Geometry: final body of the model. Coordinates: model frame, mm. A direction names the side the tool comes from. Coordinates: 2 decimals unless noted, no trailing zeros. Loops run counter-clockwise (first coordinate to the right, second up) from the corner with the lowest first, then second, coordinate; pieces in that order, holes last. Notation, with made-up numbers: (33.25, 41) -> (92.25, 41) arc R17 cw to (92.25, 64) -> close; hole circle Ø1 at (-27, 34.25). An arc over 180 degrees is marked (long way). One line per item, written item: value. Start each with the question number.
Item 1: Contact query for flat-ended pins moving along their axis: pin 1 Ø13 at (x, y) = (163.5, 44) entering from -Z; pin 2 Ø21 at (x, z) = (392.5, -577.5) entering from +Y; pin 3 Ø21.5 at (x, z) = (218, 289) entering from +Y; pin 4 Ø21 at (x, y) = (384, 408) entering from +Z. Output: stop coordinate, or through.
Item 2: Section query C-C on z = 231.5. Return loops of the section in (x, y).
Item 3: Section query B-B on z = -418. Return loops of the section in (x, y), then the cut area to 3 significant figures.
Item 4: Set-up query: faces 5 (the flat face through (198, 404, -399.91)), 6 (the flat face through (11, 387.823, 144)), 7 (the flat face through (11, 49, 99.89)), 8 (the flat face through (12, 394.98, -375)), 9 (the flat face through (198, 394.98, -259)). Return all of +Z, -Z, +X, -X, +Y, -Y with unobstructed straight access to the full face (end or side cutting, diameter ignored); none if empty.
Item 5: Mould query, pull axis X, two halves, no side actions, for faces 1 (the flat face through (402, 405, -259)), 2 (the flat face through (389, 414.065, -501)), 3 (the flat face through (342.591, 227, 120)), 4 (the flat face through (198, 35.935, 122)). Classes: +X half, -X half, draft (parallel to the pull), parting line (faces both ways), or undercut.
Item 6: Section query A-A on y = 313. Return loops of the section in (x, z) (3 decimals).
Item 7: Ray query, probe 1 along Z at (x, y) = (291, 55); probe 2 along Z at (x, y) = (364, 289) (3 decimals); probe 3 along X at (y, z) = (56, 244.5). Return the intervals inside material, ascending. Write a range as from..to.
Item 8: Section query D-D on x = 353.5. Return loops of the section in (y, z) (3 decimals), then the cut area to 3 significant figures.
from build123d import *

# Parameters (mm, degrees)
SKETCH2_W                       = 400
SKETCH2_H                       = 450
BOSS_EXTRUDE1_DEPTH             = 30
SKETCH3_W                       = 40
SKETCH3_H                       = 50
BOSS_EXTRUDE2_DEPTH             = 400
SKETCH4_W                       = 40
SKETCH4_H                       = 40
BOSS_EXTRUDE3_DEPTH             = 600
SKETCH5_W                       = 40.556580032
SKETCH5_H                       = 28.62817414
SKETCH5_W_2                     = 47.713623567
BOSS_EXTRUDE4_DEPTH             = 402
SKETCH6_W                       = 42.94226121
SKETCH6_H                       = 26.242492962
SKETCH6_W_2                     = 42.942261211
BOSS_EXTRUDE5_DEPTH             = 402
SKETCH7_W                       = 40.556580032
SKETCH7_H                       = 19.085449427
SKETCH7_W_2                     = 50.099304746
SKETCH7_W_3                     = 42.94226121
SKETCH7_W_4                     = 44.71367334
BOSS_EXTRUDE6_DEPTH             = 402
BOSS_EXTRUDE7_REACH             = 816.236
SKETCH8_W                       = 21.611464792
SKETCH8_H                       = 67.92174649
SKETCH8_H_2                     = 58.65969015
BOSS_EXTRUDE7_DIRECTION_2_DEPTH = 2
BOSS_EXTRUDE8_REACH             = 816.236
SKETCH9_W                       = 23.109912939
SKETCH9_H                       = 42.918409744
SKETCH9_H_2                     = 49.521242012


with BuildPart() as part:
    # Sketch2 → Boss-Extrude1 (new body)
    with BuildSketch(Plane.XY):
        with Locations((200, 225)):
            Rectangle(SKETCH2_W, SKETCH2_H)
    extrude(amount=BOSS_EXTRUDE1_DEPTH)

    # Sketch3 → Boss-Extrude2 (add)
    with BuildSketch(Plane.XY.offset(30)):
        with Locations((43, 401)):
            Rectangle(SKETCH3_W, SKETCH3_H)
        with Locations((357, 401)):
            Rectangle(SKETCH3_W, SKETCH3_H)
        with Locations((357, 49)):
            Rectangle(SKETCH3_W, SKETCH3_H)
        with Locations((43, 49)):
            Rectangle(SKETCH3_W, SKETCH3_H)
    extrude(amount=BOSS_EXTRUDE2_DEPTH)

    # Sketch4 → Boss-Extrude3 (add)
    with BuildSketch(Plane(origin=(0, 0, 0), x_dir=(-1, 0, 0), z_dir=(0, 0, -1))):
        with Locations((-356, 406)):
            Rectangle(SKETCH4_W, SKETCH4_H)
        with Locations((-44, 406)):
            Rectangle(SKETCH4_W, SKETCH4_H)
    extrude(amount=BOSS_EXTRUDE3_DEPTH)

    # Sketch5 → Boss-Extrude4 (add)
    with BuildSketch(Plane(origin=(0, 0, 0), x_dir=(0, 0, -1), z_dir=(1, 0, 0))):
        with Locations((-144.025393122, 402.136827493)):
            Rectangle(SKETCH5_W, SKETCH5_H)
        with Locations((-280.009220289, 402.136827493)):
            Rectangle(SKETCH5_W_2, SKETCH5_H)
    extrude(amount=BOSS_EXTRUDE4_DEPTH)

    # Sketch6 → Boss-Extrude5 (add)
    with BuildSketch(Plane(origin=(0, 0, 0), x_dir=(0, 0, -1), z_dir=(1, 0, 0))):
        with Locations((-280.009220288, 49.056013096)):
            Rectangle(SKETCH6_W, SKETCH6_H)
        with Locations((-121.361421928, 49.056013096)):
            Rectangle(SKETCH6_W_2, SKETCH6_H)
    extrude(amount=BOSS_EXTRUDE5_DEPTH)

    # Sketch7 → Boss-Extrude6 (add)
    with BuildSketch(Plane(origin=(0, 0, 0), x_dir=(0, 0, -1), z_dir=(1, 0, 0))):
        with Locations((259.15472602, 404.522508672)):
            Rectangle(SKETCH7_W, SKETCH7_H)
        with Locations((374.86026317, 404.522508672)):
            Rectangle(SKETCH7_W_2, SKETCH7_H)
        with Locations((501.301365623, 404.522508672)):
            Rectangle(SKETCH7_W_3, SKETCH7_H)
        with Locations((577.64316333, 404.522508672)):
            Rectangle(SKETCH7_W_4, SKETCH7_H)
    extrude(amount=BOSS_EXTRUDE6_DEPTH)

    # Sketch8 → Boss-Extrude7 (add, up to next)
    with BuildSketch(Plane(origin=(0, 74, 0), x_dir=(1, 0, 0), z_dir=(0, 1, 0)), mode=Mode.PRIVATE) as boss_extrude7_sk1:
        with Locations((41.856325516, -134.973838063)):
            Rectangle(SKETCH8_W, SKETCH8_H)
    boss_extrude7_tool1 = extrude(boss_extrude7_sk1.sketch, amount=BOSS_EXTRUDE7_REACH, mode=Mode.PRIVATE) - part.part
    # Sketch8 → Boss-Extrude7 (add, up to next)
    with BuildSketch(Plane(origin=(0, 74, 0), x_dir=(1, 0, 0), z_dir=(0, 1, 0)), mode=Mode.PRIVATE) as boss_extrude7_sk2:
        with Locations((41.856325516, -284.710415551)):
            Rectangle(SKETCH8_W, SKETCH8_H_2)
    boss_extrude7_tool2 = extrude(boss_extrude7_sk2.sketch, amount=BOSS_EXTRUDE7_REACH, mode=Mode.PRIVATE) - part.part
    add(boss_extrude7_tool1.solids().sort_by_distance((41.856326, 74, 134.973838))[0])
    add(boss_extrude7_tool2.solids().sort_by_distance((41.856326, 74, 284.710416))[0])

    # Sketch8 → Boss-Extrude7 direction 2 (add)
    with BuildSketch(Plane(origin=(0, 74, 0), x_dir=(1, 0, 0), z_dir=(0, 1, 0))):
        with Locations((41.856325516, -134.973838063)):
            Rectangle(SKETCH8_W, SKETCH8_H)
        with Locations((41.856325516, -284.710415551)):
            Rectangle(SKETCH8_W, SKETCH8_H_2)
    extrude(amount=-BOSS_EXTRUDE7_DIRECTION_2_DEPTH)

    # Sketch9 → Boss-Extrude8 (add, up to next)
    with BuildSketch(Plane.XZ.offset(-376), mode=Mode.PRIVATE) as boss_extrude8_sk1:
        with Locations((354.146322372, 280.024195097)):
            Rectangle(SKETCH9_W, SKETCH9_H)
    boss_extrude8_tool1 = extrude(boss_extrude8_sk1.sketch, amount=BOSS_EXTRUDE8_REACH, mode=Mode.PRIVATE) - part.part
    # Sketch9 → Boss-Extrude8 (add, up to next)
    with BuildSketch(Plane.XZ.offset(-376), mode=Mode.PRIVATE) as boss_extrude8_sk2:
        with Locations((354.146322372, 119.905512592)):
            Rectangle(SKETCH9_W, SKETCH9_H_2)
    boss_extrude8_tool2 = extrude(boss_extrude8_sk2.sketch, amount=BOSS_EXTRUDE8_REACH, mode=Mode.PRIVATE) - part.part
    add(boss_extrude8_tool1.solids().sort_by_distance((354.146322, 376, 280.024195))[0])
    add(boss_extrude8_tool2.solids().sort_by_distance((354.146322, 376, 119.905513))[0])


solid = part.part
Reply:
1. pin 1: stops at z = 0
1. pin 2: stops at y = 414.07
1. pin 3: stops at y = 416.45
1. pin 4: stops at z = 430
2. outline: (23, 24) -> (63, 24) -> (63, 74) -> (23, 74) -> close; (23, 376) -> (63, 376) -> (63, 426) -> (23, 426) -> close; (337, 24) -> (377, 24) -> (377, 74) -> (337, 74) -> close; (337, 376) -> (377, 376) -> (377, 426) -> (337, 426) -> close
3. outline: (24, 386) -> (64, 386) -> (64, 426) -> (24, 426) -> close; (336, 386) -> (376, 386) -> (376, 426) -> (336, 426) -> close
3. area: 3,200 mm²
4. face 5: +Y, -Y
4. face 6: +Z, -X
4. face 7: -X, +Y, -Y
4. face 8: -Z, -X, -Y
4. face 9: -Z, -Y
5. face 1: +X half
5. face 2: draft
5. face 3: undercut
5. face 4: undercut
6. outline: (0, 0) -> (400, 0) -> (400, 30) -> (0, 30) -> close; (31.051, 101.013) -> (52.662, 101.013) -> (52.662, 168.935) -> (31.051, 168.935) -> close; (31.051, 255.381) -> (52.662, 255.381) -> (52.662, 314.04) -> (31.051, 314.04) -> close; (342.591, 95.145) -> (365.701, 95.145) -> (365.701, 144.666) -> (342.591, 144.666) -> close; (342.591, 258.565) -> (365.701, 258.565) -> (365.701, 301.483) -> (342.591, 301.483) -> close
7. probe 1: z = 0..30, 99.89..142.83, 258.54..301.48
7. probe 2: z = 0..30, 95.145..144.666, 258.565..301.483
7. probe 3: x = 23..63, 337..377
8. outline: (0, 0) -> (386, 0) -> (386, -600) -> (426, -600) -> (426, 0) -> (450, 0) -> (450, 30) -> (426, 30) -> (426, 430) -> (376, 430) -> (376, 301.483) -> (74, 301.483) -> (74, 430) -> (24, 430) -> (24, 30) -> (0, 30) -> close; hole (74, 30) -> (376, 30) -> (376, 95.145) -> (74, 95.145) -> close; hole (74, 144.666) -> (376, 144.666) -> (376, 258.565) -> (74, 258.565) -> close
8. area: 105,000 mm²
